Geometry: see drawing. Coordinates: mm, zero at the bounding-box minimum. A direction names the side the tool comes from. Give positions to 0.01 mm unless a question says otherwise; leave off trailing zeros. Write each loop counter-clockwise with the first axis right and the second up, starting at its lowest first coordinate (ties: lowest second). Pieces come first, ordered by that corner, then holes. Notation, with made-up numbers: M -26.75,1 L -16.75,1 A25 cw -16.75,20 Z; hole C 73.25,66.5 d7. An arc over 180 degrees is marked long. Use one line per item in the form item = value. Start each with the question number.
Item 1: Section query C-C on x = 7.25. Return loops of the section in (y, z).
Item 2: Access query for the marked faces 1 and 2. Directions: +Z, -Z, +X, -X, +Y, -Y. A direction counts if a zero-diameter tool reaches every point of the face in a straight line with its end or side. Return the directions, or none.
Item 3: Section query B-B on z = 1.2. Return loops of the section in (x, y) (3 decimals), then the cut area to 3 significant figures.
Item 4: Material intervals for line 1 along Z through (x, y) = (2.8, 0.4) (3 decimals); line 2 along Y through (x, z) = (0.5, 1.2) (3 decimals); line 3 along Y through (x, z) = (6.5, 0.7), sorted ascending. Write a range as from..to.
Item 5: Section query A-A on x = 8.8. Return loops of the section in (y, z) (3 decimals).
Item 6: Contact query for flat-ended pins moving along their axis: P1, Ø3, axis at x = 7, z = 1.5, coming from the +Y side; P2, Ø1, axis at y = 7.5, z = 4.5, coming from the +X side. Output: stop coordinate, or through.
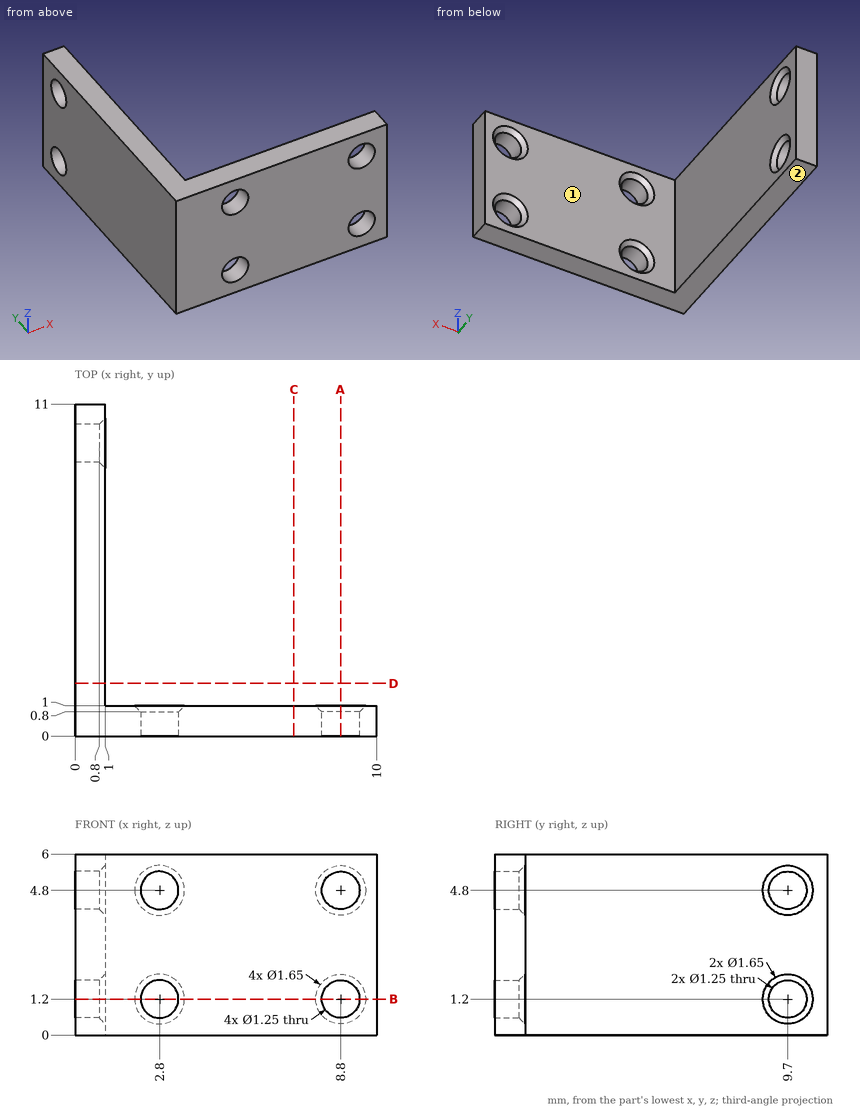
Answer sheet:
q1.outline = M 0,0 L 1,0 L 1,6 L 0,6 Z
q2.face_1 = +Z, -Z, +X, +Y
q2.face_2 = -Z, +X, -X, +Y, -Y
q3.outline = M 0,0 L 2.175,0 L 2.175,0.8 L 1.975,1 L 1,1 L 1,8.875 L 0.8,9.075 L 0,9.075 Z; M 0,10.325 L 0.8,10.325 L 1,10.525 L 1,11 L 0,11 Z; M 3.425,0 L 8.175,0 L 8.175,0.8 L 7.975,1 L 3.625,1 L 3.425,0.8 Z; M 9.425,0 L 10,0 L 10,1 L 9.625,1 L 9.425,0.8 Z
q3.area = 16.1 mm2
q4.line_1 = 0..0.575, 1.825..4.175, 5.425..6
q4.line_2 = 0..9.075, 10.325..11
q4.line_3 = 0..1
q5.outline = M 0,0 L 1,0 L 1,0.375 L 0.8,0.575 L 0,0.575 Z; M 0,1.825 L 0.8,1.825 L 1,2.025 L 1,3.975 L 0.8,4.175 L 0,4.175 Z; M 0,5.425 L 0.8,5.425 L 1,5.625 L 1,6 L 0,6 Z
q6.P1 = 1
q6.P2 = 1
